```python
from build123d import *

# Parameters (mm, degrees)
SKETCH_R           = 70
SKETCH_R_2         = 2.5
PAD_DEPTH          = 10
SKETCH002_R        = 7
POCKET_DEPTH       = 11
SKETCH003_R        = 1.5
POCKET001_DEPTH    = 20
POCKET002_DEPTH    = 12
SKETCH005_R        = 1.5
POCKET003_DEPTH    = 12
POCKET004_DEPTH    = 12
SKETCH007_R        = 1.5
POCKET005_DEPTH    = 20
POCKET006_DEPTH    = 5
POLARPATTERN_COUNT = 6
SKETCH009_R        = 6.5
POCKET007_DEPTH    = 20
POCKET008_DEPTH    = 4


with BuildPart() as part:
    # Sketch → Pad (new body)
    with BuildSketch(Plane.XY):
        Circle(SKETCH_R)
        with Locations((-38.6, 51.05)):
            Circle(SKETCH_R_2, mode=Mode.SUBTRACT)
        with Locations((38.6, 51.05)):
            Circle(SKETCH_R_2, mode=Mode.SUBTRACT)
        with Locations((-38.6, -51.05)):
            Circle(SKETCH_R_2, mode=Mode.SUBTRACT)
        with Locations((38.6, -51.05)):
            Circle(SKETCH_R_2, mode=Mode.SUBTRACT)
    extrude(amount=PAD_DEPTH)

    # Sketch001 → Revolution (revolve)
    with BuildSketch(Plane.XZ):
        Polygon((0, 10), (46.5, 10), (42.5, 17), (0, 17), align=None)
    revolve(axis=Axis((0, 0, 0), (0, 0, 1)))

    # Sketch002 (on Face3 of Revolution) → Pocket (cut)
    with BuildSketch(Plane.XY.offset(10)):
        with Locations((0, -58)):
            Circle(SKETCH002_R)
        with Locations((-50.2294734195, 29)):
            Circle(SKETCH002_R)
        with Locations((-50.2294734195, -29)):
            Circle(SKETCH002_R)
        with Locations((50.2294734195, -29)):
            Circle(SKETCH002_R)
        with Locations((0, 58)):
            Circle(SKETCH002_R)
    extrude(amount=-POCKET_DEPTH, mode=Mode.SUBTRACT)

    # Sketch003 (on Face14 of Pocket) → Pocket001 (cut)
    with BuildSketch(Plane.XY.offset(17)):
        with Locations((0, 27.5)):
            Circle(SKETCH003_R)
        with Locations((23.8156986041, 13.75)):
            Circle(SKETCH003_R)
        with Locations((23.8156986041, -13.75)):
            Circle(SKETCH003_R)
        with Locations((0, -27.5)):
            Circle(SKETCH003_R)
        with Locations((-23.8156986041, -13.75)):
            Circle(SKETCH003_R)
        with Locations((-23.8156986041, 13.75)):
            Circle(SKETCH003_R)
    extrude(amount=-POCKET001_DEPTH, mode=Mode.SUBTRACT)

    # Sketch004 (on Face3 of Pocket001) → Pocket002 (cut)
    with BuildSketch(Plane.XY.offset(10)):
        with BuildLine():
            Line((60.4572715312, 8.1323563009), (68.8940277881, 12.3940685462))
            ThreePointArc((68.8940277881, 12.3940685462), (62.4810072916, 31.5614278483), (50.8589261605, 48.0975012843))
            Line((42.4221699036, 43.835789039), (50.8589261605, 48.0975012843))
            Line((42.4221699036, 43.835789039), (60.4572715312, 8.1323563009))
        make_face()
    extrude(amount=-POCKET002_DEPTH, mode=Mode.SUBTRACT)

    # Sketch005 (on Face4 of Pocket002) → Pocket003 (cut)
    with BuildSketch(Plane.XY.offset(10)):
        with Locations((62.5, 0)):
            Circle(SKETCH005_R)
    extrude(amount=-POCKET003_DEPTH, mode=Mode.SUBTRACT)

    # Sketch006 (on Face4 of Pocket003) → Pocket004 (cut)
    with BuildSketch(Plane.XY.offset(10)):
        Polygon((35.8450802819, 39.1130364404), (38.5228377372, 40.4656690625), (41.002664211, 35.556447061), (38.3249067556, 34.2038144389), align=None)
        Polygon((50.2731615839, 10.5502902499), (52.9509190393, 11.902922872), (55.4307455131, 6.9937008705), (52.7529880577, 5.6410682484), align=None)
    extrude(amount=-POCKET004_DEPTH, mode=Mode.SUBTRACT)

    # Sketch007 (on Face7 of Pocket004) → Pocket005 (cut)
    with BuildSketch(Plane(origin=(51.4397207174, 25.9840726699, 0), x_dir=(-0.4508775407, 0.8925858185, 0), z_dir=(0.8925858185, 0.4508775407, 0))):
        with Locations((-16, 5)):
            Circle(SKETCH007_R)
        with Locations((16, 5)):
            Circle(SKETCH007_R)
    extrude(amount=-POCKET005_DEPTH, mode=Mode.SUBTRACT)

    # Sketch008 (on Face2 of Pocket005) → Pocket006 (cut)
    with BuildSketch(Plane(origin=(0, 0, 0), x_dir=(1, 0, 0), z_dir=(0, 0, -1))):
        Polygon((-1.5588457268, 24.8), (1.5588457268, 24.8), (3.1176914536, 27.5), (1.5588457268, 30.2), (-1.5588457268, 30.2), (-3.1176914536, 27.5), align=None)
    pocket006 = extrude(amount=-POCKET006_DEPTH, mode=Mode.SUBTRACT)

    # PolarPattern: Pocket006 ×6 about axis
    polarpattern_axis = Axis((0, 0, 0), (0, 0, -1))
    for i in range(1, POLARPATTERN_COUNT):
        add(pocket006.rotate(polarpattern_axis, i * 360 / POLARPATTERN_COUNT), mode=Mode.SUBTRACT)

    # Sketch009 (on Face73 of PolarPattern) → Pocket007 (cut)
    with BuildSketch(Plane.XY.offset(17)):
        Circle(SKETCH009_R)
    extrude(amount=-POCKET007_DEPTH, mode=Mode.SUBTRACT)

    # Sketch010 (on Face2 of Pocket007) → Pocket008 (cut)
    with BuildSketch(Plane(origin=(0, 0, 0), x_dir=(1, 0, 0), z_dir=(0, 0, -1))):
        Polygon((65.2, -1.5588457268), (65.2, 1.5588457268), (62.5, 3.1176914536), (59.8, 1.5588457268), (59.8, -1.5588457268), (62.5, -3.1176914536), align=None)
    extrude(amount=-POCKET008_DEPTH, mode=Mode.SUBTRACT)


solid = part.part
```
Source: CAD feature listing. Evaluate the final solid. Frame: model axes, mm. A direction names the side the tool comes from. Coordinates: 2 decimals unless noted, no trailing zeros. Loops run counter-clockwise (first coordinate to the right, second up) from the corner with the lowest first, then second, coordinate; pieces in that order, holes last. Notation, with made-up numbers: M 13.5,28.25 L 45.5,28.25 A20 cw 45.5,61.25 Z; hole C 6,48.25 d10. An arc over 180 degrees is marked long. Use a Markdown table: item, result. Add a question column.
Q1. Access query for faces 5 (the flat face through (-17, -46, 10)), 6 (the cylindrical face through (22.317, 13.816, 11.084)), 7 (the flat face through (-24, -12, 5)). Directions: +Z, -Z, +X, -X, +Y, -Y. A direction counts if a zero-diameter tool reaches every point of the face in a straight line with its end or side. Return the directions, or none.
Q2. Section query B-B, the plane y = -33. State how many separate pieces and enclosed holes the cut face has, and give its area (3 significant figures).
Q3. Draft query along Y for faces 1 (the cylindrical face through (-63.69, -29.04, 4.93)), 2 (the flat face through (-1, -15, 0)), 3 (the flat face through (24, 11.05, 2)), 4 (the cylindrical face through (22.317, -13.684, 11.084)). Return one class per face: pulls with the +Y half, pulls with the -Y half, needs draft (parallel to the pull), parting line crosses it, or undercut.
Q4. Section query A-A, the plane y = 58. Return loops of the section in (x, z).
Q5. Material intervals for L1, parallel to Y at x = 0, z = 3.75; L2, parallel to Y at x = 38.6, z = 2.75; L3, parallel to X at y = -13, z = 4, sorted ascending.
Q6. First-contact query: pin 1 (2.5 mm diameter, centred on x = 0.5, z = 3, fed in from -Y); pin 2 (2.5 mm diameter, centred on x = -23.82, y = -13.75, fed in from -Z); pin 3 (3.5 mm diameter, centred on y = -0.5, z = 3, fed in from -X); pin 4 (5 mm diameter, centred on y = 18, z = 13.5, fed in from -X). Flat tips, straight axial feed; report the tip coordinate or a pass-through.
Result:
| question | item | result |
|---|---|---|
| 1 | face 5 | +Z |
| 1 | face 6 | +Z, -Z |
| 1 | face 7 | -Z |
| 2 | separate pieces | 3 |
| 2 | enclosed holes | 0 |
| 2 | area | 1,420 mm2 |
| 3 | face 1 | parting line crosses it |
| 3 | face 2 | needs draft |
| 3 | face 3 | undercut |
| 3 | face 4 | undercut |
| 4 | outline | M -39.19,0 L -7,0 L -7,10 L -39.19,10 Z; M 7,0 L 39.19,0 L 39.19,10 L 7,10 Z |
| 5 | L1 | y = -70 to -65, -51 to -30.2, -24.8 to -6.5, 6.5 to 24.8, 30.2 to 51, 65 to 70 |
| 5 | L2 | y = -58.4 to -53.55, -48.55 to 34.34, 40.31 to 48.55, 53.55 to 58.4 |
| 5 | L3 | x = -68.78 to -26.5, -21.13 to 21.13, 26.5 to 68.78 |
| 6 | pin 1 | stops at y = -70 |
| 6 | pin 2 | passes through |
| 6 | pin 3 | stops at x = -70 |
| 6 | pin 4 | stops at x = -42.56 |
